```python
from build123d import *

# Parameters (mm, degrees)
SKETCH1_W           = 28
SKETCH1_H           = 8
BOSS_EXTRUDE1_DEPTH = 1
SKETCH2_W           = 28
SKETCH2_H           = 1
BOSS_EXTRUDE2_DEPTH = 30
SKETCH3_R           = 1.65
CUT_EXTRUDE1_DEPTH  = 1
CHAMFER1_SIZE       = 4
SKETCH4_W           = 3.3
SKETCH4_H           = 27
SKETCH4_H_2         = 25
CUT_EXTRUDE2_DEPTH  = 10


with BuildPart() as part:
    # Sketch1 → Boss-Extrude1 (new body)
    with BuildSketch(Plane.XY):
        Rectangle(SKETCH1_W, SKETCH1_H)
    extrude(amount=BOSS_EXTRUDE1_DEPTH)

    # Sketch2 → Boss-Extrude2 (add)
    with BuildSketch(Plane(origin=(0, 0, 0), x_dir=(-1, 0, 0), z_dir=(0, 0, -1))):
        with Locations((0, 3.5)):
            Rectangle(SKETCH2_W, SKETCH2_H)
    extrude(amount=BOSS_EXTRUDE2_DEPTH)

    # Sketch3 → Cut-Extrude1 (cut)
    with BuildSketch(Plane.XY.offset(1)):
        with Locations((-7, -1.5)):
            Circle(SKETCH3_R)
        with Locations((7, -1.5)):
            Circle(SKETCH3_R)
    extrude(amount=-CUT_EXTRUDE1_DEPTH, mode=Mode.SUBTRACT)

    # Chamfer1
    chamfer1_edges = [part.edges().sort_by_distance(p)[0] for p in [
        (14, -4, 0.5),
        (-14, -4, 0.5),
    ]]
    chamfer(chamfer1_edges, length=CHAMFER1_SIZE)

    # Sketch4 → Cut-Extrude2 (cut)
    with BuildSketch(Plane(origin=(0, 4, 0), x_dir=(1, 0, 0), z_dir=(0, 1, 0))):
        with Locations((11.5, 15)):
            Rectangle(SKETCH4_W, SKETCH4_H)
        with Locations((-11.5, 16)):
            Rectangle(SKETCH4_W, SKETCH4_H_2)
    extrude(amount=-CUT_EXTRUDE2_DEPTH, mode=Mode.SUBTRACT)


solid = part.part
```
For this review, take the finished solid that the model builds, in its own axes (mm). A direction names the side the tool comes from. Coordinates: 2 decimals unless noted, no trailing zeros. Write each loop counter-clockwise with the first axis right and the second up, starting at its lowest first coordinate (ties: lowest second). Pieces come first, ordered by that corner, then holes. Notation, with made-up numbers: (-15.75, -37) - (30.25, -37) arc R22 cw to (30.25, 1) - close; hole circle Ø5 at (21, 56.5). An arc over 180 degrees is marked (long way). Put each result on its own line as item: value.
1. Add section B-B, the plane y = -1.5. Give the boundary of the cut face in (x, z), then the cut area to 3 significant figures.
Values found:
outline: (-12.5, 0) - (-8.65, 0) - (-8.65, 1) - (-12.5, 1) - close; (-5.35, 0) - (5.35, 0) - (5.35, 1) - (-5.35, 1) - close; (8.65, 0) - (12.5, 0) - (12.5, 1) - (8.65, 1) - close
area: 18.4 mm²
2. Machinability: for faces 1 (the flat face through (-13.15, 3.5, -15.8)), 2 (the flat face through (-14, 3.3, -13.3)), which of the approach directions +Z, -Z, +X, -X, +Y, -Y give a long, thin tool a straight path to every point of the face, cutting with its end or side? Answer none if there is none.
Values found:
face 1: +Y, -Y
face 2: +Z, -Z, -X, +Y, -Y
3. Add section A-A, the plane x = -10.5. Give the boundary of the cut face in (y, z), then the cut area to 3 significant figures.
Values found:
outline: (-3.5, 0) - (3, 0) - (3, -3.5) - (4, -3.5) - (4, 1) - (-3.5, 1) - close; (3, -30) - (4, -30) - (4, -28.5) - (3, -28.5) - close
area: 12.5 mm²
4. Add section D-D, the plane x = 11.25. Give the boundary of the cut face in (y, z).
Values found:
outline: (-2.75, 0) - (3, 0) - (3, -1.5) - (4, -1.5) - (4, 1) - (-2.75, 1) - close; (3, -30) - (4, -30) - (4, -28.5) - (3, -28.5) - close
5. Add section C-C, the plane z = -15. Give the boundary of the cut face in (x, y), then the cut area to 3 significant figures.
Values found:
outline: (-14, 3) - (-13.15, 3) - (-13.15, 4) - (-14, 4) - close; (-9.85, 3) - (9.85, 3) - (9.85, 4) - (-9.85, 4) - close; (13.15, 3) - (14, 3) - (14, 4) - (13.15, 4) - close
area: 21.4 mm²
6. Wall thickness on probe 1 along X at (y, z) = (3.25, -9); probe 2 along Y at (x, z) = (7, 0.2); probe 3 along Y at (x, z) = (7.25, -13.5): over which ranges is each line inside the solid? List them lowest first.
Values found:
probe 1: -14 to -13.15, -9.85 to 9.85, 13.15 to 14
probe 2: -4 to -3.15, 0.15 to 4
probe 3: 3 to 4
7. For pin 1 (4 mm diameter, centred on x = 6.5, y = 0, fed in from +Z); pin 2 (14 mm diameter, centred on x = 3.5, z = -16, fed in from -Y); pin 3 (4.5 mm diameter, centred on x = -7, y = -1.5, fed in from -Z), all flat-tipped, find the tip position at first contact; note any pin that passes through.
Values found:
pin 1: z = 1
pin 2: y = 3
pin 3: z = 0
8. Mouldability with a two-part tool opening along X and no side actions: class faces 3 (the flat face through (-12, -2, 0.5)), 4 (the flat face through (0, 3, -15)), 5 (the flat face through (11.5, 3.5, -28.5)) as released by +X, released by -X, zero draft, split by the parting line, or undercut.
Values found:
face 3: released by -X
face 4: zero draft
face 5: undercut
